Geometry check sheet. Reference: the model listing, model coordinates, mm. Face numbers are marked on the shaded views. A direction names the side the tool comes from. Give positions to 0.01 mm unless a question says otherwise; leave off trailing zeros. Write each loop counter-clockwise with the first axis right and the second up, starting at its lowest first coordinate (ties: lowest second). Pieces come first, ordered by that corner, then holes. Notation, with made-up numbers: M -35.5,58.25 L -25.5,58.25 A12 ccw -25.5,65.25 Z; hole C 10.25,-7 d6. An arc over 180 degrees is marked long. One line per item, written item: value. Start each with the question number.
1. Release check for a two-part mould opening along Z. For the marked faces 3, 4, 5 and 6 record: pulls with the +Z half, pulls with the -Z half, needs draft (parallel to the pull), parting line crosses it, or undercut.
2. Cross-section at B-B on x = 5. Record the cut outline in (y, z).
3. Cross-section at D-D on x = 8.5. Record the cut outline in (y, z).
4. Gauge pin test, flat ends, axial feed: pin 1 (0.9 mm diameter, centred on x = 7, z = 0.5, fed in from -Y); pin 2 (2.5 mm diameter, centred on x = 6.5, y = 4, fed in from +Z); pin 3 (0.9 mm diameter, centred on x = 3.5, y = 13, fed in from +Z); pin 4 (3 mm diameter, centred on x = 5, z = -20, fed in from -Y). Record the tip position at first contact, or that the pin passes through.
5. Tool access check on the marked faces 1 and 2. Record the directions out of +Z, -Z, +X, -X, +Y, -Y that give a thin tool (end or side, any length) a straight path to the whole face; none if there is none.
6. Cross-section at C-C on y = 6. Record the cut outline in (x, z).
7. Cross-section at A-A on z = -20. Record the cut outline in (x, y).
8. Scan lines: line 1 (X direction, y = 14.45, z = -20); line 2 (Z direction, x = 2.25, y = 1.75); line 3 (Y direction, x = 8.5, z = -12.25). Record each from-to range of solid material in increasing order.
from build123d import *

# Parameters (mm, degrees)
BOSS_EXTRUDE2_DEPTH = 10
SKETCH2_R           = 2
CUT_EXTRUDE9_DEPTH  = 3


with BuildPart() as part:
    # Sketch1 → Boss-Extrude2 (new body)
    with BuildSketch(Plane(origin=(0, 0, 0), x_dir=(0, 0, -1), z_dir=(1, 0, 0))):
        Polygon((0, 0), (0, 7.6), (-1.8, 7.6), (-1.8, 4.921680622), (-4.55, 7.671680622), (-4.55, 12.5), (-1.8, 15.25), (-1.8, 12.4), (0, 12.4), (0, 15.25), (25, 15.25), (25, 13.25), (6, 13.25), (2, 9.25), (2, 0), align=None)
    extrude(amount=BOSS_EXTRUDE2_DEPTH)

    # Sketch2 → Cut-Extrude9 (cut)
    with BuildSketch(Plane(origin=(0, 15.25, 0), x_dir=(1, 0, 0), z_dir=(0, 1, 0))):
        with Locations(Location((5, 20, 0), (0, 0, 270))):
            Circle(SKETCH2_R)
    extrude(amount=-CUT_EXTRUDE9_DEPTH, mode=Mode.SUBTRACT)


solid = part.part
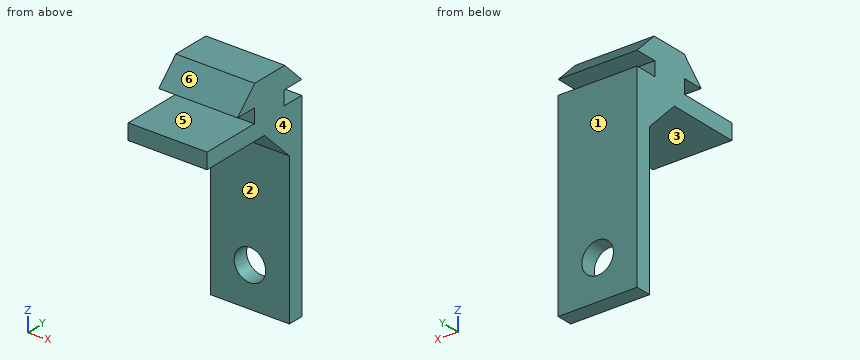
Report:
1. face 3: pulls with the -Z half
1. face 4: needs draft
1. face 5: undercut
1. face 6: pulls with the +Z half
2. outline: M 0,-2 L 9.25,-2 L 13.25,-6 L 13.25,-18 L 15.25,-18 L 15.25,0 L 12.4,0 L 12.4,1.8 L 15.25,1.8 L 12.5,4.55 L 7.67,4.55 L 4.92,1.8 L 7.6,1.8 L 7.6,0 L 0,0 Z; M 13.25,-25 L 15.25,-25 L 15.25,-22 L 13.25,-22 Z
3. outline: M 0,-2 L 9.25,-2 L 13.25,-6 L 13.25,-25 L 15.25,-25 L 15.25,0 L 12.4,0 L 12.4,1.8 L 15.25,1.8 L 12.5,4.55 L 7.67,4.55 L 4.92,1.8 L 7.6,1.8 L 7.6,0 L 0,0 Z
4. pin 1: stops at y = 7.6
4. pin 2: stops at z = 2.13
4. pin 3: stops at z = 4.5
4. pin 4: passes through
5. face 1: +Z, -Z, +X, -X, +Y
5. face 2: -Z, +X, -X, -Y
6. outline: M 0,-2 L 10,-2 L 10,0 L 0,0 Z; M 0,1.8 L 10,1.8 L 10,2.88 L 0,2.88 Z
7. outline: M 0,13.25 L 3,13.25 L 3,15.25 L 0,15.25 Z; M 7,13.25 L 10,13.25 L 10,15.25 L 7,15.25 Z
8. line 1: x = 0 to 3, 7 to 10
8. line 2: z = -2 to 0
8. line 3: y = 13.25 to 15.25
